Here's how the part is built. I have some questions about the finished solid (model axes, mm). Coordinates: 2 decimals unless noted, no trailing zeros. Loops run counter-clockwise (first coordinate to the right, second up) from the corner with the lowest first, then second, coordinate; pieces in that order, holes last. Notation, with made-up numbers: M -21,32 L -4,32 A37 ccw -4,68 Z; hole C -2,-14.75 d11. An arc over 180 degrees is marked long. Use CSV: the item, a comma, the result in double quotes. Start each with the question number.
Q1. For pin 1 Ø5 at (x, y) = (-190.5, 682.38) entering from +Z; pin 2 Ø1.9 at (x, z) = (173.5, 2) entering from +Y, each with a flat end and sliding along its axis, tell me the tip position at first contact or that it passes through.
Q2. If we section it at D-D (z = 3.25): State how many separate pieces and enclosed holes the cut face has, and give its area (3 significant figures).
Q3. Please list where these lines run through material, in increasing order: probe 1 along Y at (x, z) = (47, 0.75); probe 2 along X at (y, z) = (889, 2.5); probe 3 along X at (y, z) = (813.5, 2). Write a range as [from, to].
Q4. If we section it at B-B (x = -19): Please give me the cut outline in (y, z).
Q5. If we section it at A-A (y = 250.5): Please give me the cut outline in (x, z).
Q6. If we section it at C-C (y = 1278.5): Please give me the cut outline in (x, z), and give its area (3 significant figures).
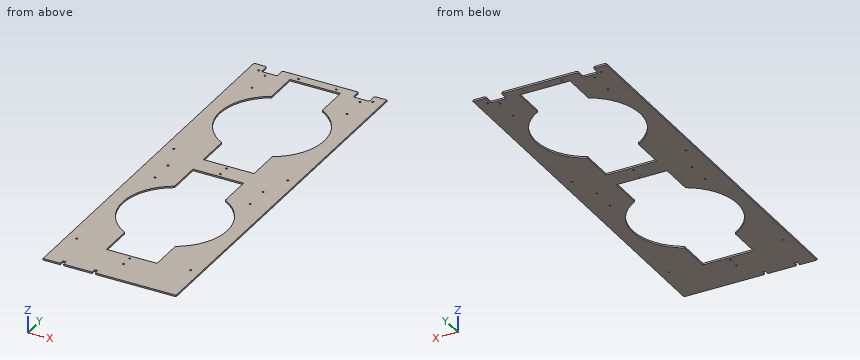
from build123d import *

# Parameters (mm, degrees)
SKETCH1_W                      = 533.4
SKETCH1_H                      = 2413
BOSS_EXTRUDE1_DEPTH            = 6.35
F_5_16_0_3125_DIAMETER_HOLE1_D = 7.9375
SKETCH6_W                      = 533.4
SKETCH6_H                      = 866.14
CUT_EXTRUDE1_DEPTH             = 7.35
SKETCH8_W                      = 63.5
SKETCH8_H                      = 38.1
CUT_EXTRUDE2_DEPTH             = 7.35
FILLET1_R                      = 6.35
F_5_16_0_3125_DIAMETER_HOLE2_D = 7.9375
SKETCH12_W                     = 13.208
SKETCH12_H                     = 19.05
CUT_EXTRUDE3_DEPTH             = 7.35
FILLET2_R                      = 3.175


with BuildPart() as part:
    # Sketch1 → Boss-Extrude1 (new body)
    with BuildSketch(Plane.XY):
        with Locations((0, 1206.5)):
            Rectangle(SKETCH1_W, SKETCH1_H)
        with BuildLine():
            Line((-101.6, 797.56), (101.6, 797.56))
            Line((101.6, 797.56), (101.6, 663.332045059))
            ThreePointArc((101.6, 663.332045059), (209.55, 480.06), (101.6, 296.787954941))
            Line((101.6, 296.787954941), (101.6, 162.56))
            Line((101.6, 162.56), (-101.6, 162.56))
            Line((-101.6, 162.56), (-101.6, 296.787954941))
            ThreePointArc((-101.6, 296.787954941), (-209.55, 480.06), (-101.6, 663.332045059))
            Line((-101.6, 663.332045059), (-101.6, 797.56))
        make_face(mode=Mode.SUBTRACT)
        with BuildLine():
            Line((-101.6, 1508.76), (-101.6, 1374.532045059))
            ThreePointArc((-101.6, 1374.532045059), (-209.55, 1191.26), (-101.6, 1007.987954941))
            Line((-101.6, 1007.987954941), (-101.6, 873.76))
            Line((-101.6, 873.76), (101.6, 873.76))
            Line((101.6, 873.76), (101.6, 1007.987954941))
            ThreePointArc((101.6, 1007.987954941), (209.55, 1191.26), (101.6, 1374.532045059))
            Line((101.6, 1374.532045059), (101.6, 1508.76))
            Line((101.6, 1508.76), (-101.6, 1508.76))
        make_face(mode=Mode.SUBTRACT)
        with BuildLine():
            Line((-101.6, 2219.96), (-101.6, 2085.732045059))
            ThreePointArc((-101.6, 2085.732045059), (-209.55, 1902.46), (-101.6, 1719.187954941))
            Line((-101.6, 1719.187954941), (-101.6, 1584.96))
            Line((-101.6, 1584.96), (101.6, 1584.96))
            Line((101.6, 1584.96), (101.6, 1719.187954941))
            ThreePointArc((101.6, 1719.187954941), (209.55, 1902.46), (101.6, 2085.732045059))
            Line((101.6, 2085.732045059), (101.6, 2219.96))
            Line((101.6, 2219.96), (-101.6, 2219.96))
        make_face(mode=Mode.SUBTRACT)
    extrude(amount=BOSS_EXTRUDE1_DEPTH)

    # 5/16 (0.3125) Diameter Hole1 (through all)
    with Locations(Plane.XY.offset(6.35)):
        with Locations((0, 146.685), (0, 102.235), (-228.6, 177.8), (0, 857.885), (0, 813.435), (228.6, 177.8), (-228.6, 889), (228.6, 889), (-76.2, 1524.635), (-76.2, 1569.085), (76.2, 1569.085), (76.2, 1524.635), (-228.6, 1511.3), (228.6, 1511.3)):
            Hole(F_5_16_0_3125_DIAMETER_HOLE1_D / 2)

    # Sketch6 → Cut-Extrude1 (cut, through all)
    with BuildSketch(Plane.XY.offset(6.35)):
        with Locations((0, 1979.93)):
            Rectangle(SKETCH6_W, SKETCH6_H)
    extrude(amount=-CUT_EXTRUDE1_DEPTH, mode=Mode.SUBTRACT)

    # Sketch8 → Cut-Extrude2 (cut, through all)
    with BuildSketch(Plane.XY.offset(6.35)):
        with Locations((-184.15, 1527.81)):
            Rectangle(SKETCH8_W, SKETCH8_H)
        with Locations((184.15, 1527.81)):
            Rectangle(SKETCH8_W, SKETCH8_H)
    extrude(amount=-CUT_EXTRUDE2_DEPTH, mode=Mode.SUBTRACT)

    # Fillet1
    fillet1_edges = [part.edges().sort_by_distance(p)[0] for p in [
        (-152.4, 1508.76, 3.175),
        (-215.9, 1508.76, 3.175),
        (-215.9, 1546.86, 3.175),
        (-152.4, 1546.86, 3.175),
        (152.4, 1508.76, 3.175),
        (152.4, 1546.86, 3.175),
        (215.9, 1546.86, 3.175),
        (215.9, 1508.76, 3.175),
    ]]
    fillet(fillet1_edges, radius=FILLET1_R)

    # 5/16 (0.3125) Diameter Hole2 (through all)
    with Locations(Plane.XY.offset(6.35)):
        with Locations((-190.5, 682.382045059), (-190.5, 777.632045059), (190.5, 777.632045059), (190.5, 682.382045059), (-190.5, 1393.582045059), (-190.5, 1488.832045059), (190.5, 1488.832045059), (190.5, 1393.582045059)):
            Hole(F_5_16_0_3125_DIAMETER_HOLE2_D / 2)

    # Sketch12 → Cut-Extrude3 (cut, through all)
    with BuildSketch(Plane.XY.offset(6.35)):
        with Locations((-63.5, 9.525)):
            Rectangle(SKETCH12_W, SKETCH12_H)
        with Locations((-190.5, 9.525)):
            Rectangle(SKETCH12_W, SKETCH12_H)
    extrude(amount=-CUT_EXTRUDE3_DEPTH, mode=Mode.SUBTRACT)

    # Fillet2
    fillet2_edges = [part.edges().sort_by_distance(p)[0] for p in [
        (-56.896, 19.05, 3.175),
        (-70.104, 19.05, 3.175),
        (-183.896, 19.05, 3.175),
        (-197.104, 19.05, 3.175),
    ]]
    fillet(fillet2_edges, radius=FILLET2_R)


solid = part.part
Results below:
1,pin 1,"through"
1,pin 2,"y = 1508.76"
2,separate pieces,"1"
2,enclosed holes,"22"
2,area,"448,000 mm^2"
3,probe 1,"[0, 162.56], [797.56, 873.76], [1508.76, 1546.86]"
3,probe 2,"[-266.7, -232.57], [-224.63, -101.6], [101.6, 224.63], [232.57, 266.7]"
3,probe 3,"[-266.7, -3.97], [3.97, 266.7]"
4,outline,"M 0,0 L 162.56,0 L 162.56,6.35 L 0,6.35 Z; M 797.56,0 L 873.76,0 L 873.76,6.35 L 797.56,6.35 Z; M 1508.76,0 L 1546.86,0 L 1546.86,6.35 L 1508.76,6.35 Z"
5,outline,"M -266.7,0 L -101.6,0 L -101.6,6.35 L -266.7,6.35 Z; M 101.6,0 L 266.7,0 L 266.7,6.35 L 101.6,6.35 Z"
6,outline,"M -266.7,0 L -190.53,0 L -190.53,6.35 L -266.7,6.35 Z; M 190.53,0 L 266.7,0 L 266.7,6.35 L 190.53,6.35 Z"
6,area,"967 mm^2"
